The model under review builds one solid part; all positions refer to its coordinate system, in mm. A direction names the side the tool comes from. Round coordinates to 2 decimals unless told otherwise and drop trailing zeros. Write each loop counter-clockwise with the first axis right and the second up, starting at its lowest first coordinate (ties: lowest second). Pieces come first, ordered by that corner, then holes. Notation, with made-up numbers: M 29,-2.75 L 58,-2.75 A13 cw 58,5.25 Z; hole C 12,40.25 d1. An arc over 180 degrees is marked long. Write item = value, one per line. Start each with the question number.
Item 1: Tool access review of faces 1 (the flat face through (-32, 0, -6.35)), 2 (the flat face through (32, 0, -19.05)), 3 (the flat face through (-31.572, -5.474, -15.919)): name each direction out of +Z, -Z, +X, -X, +Y, -Y from which nothing blocks a thin tool from reaching the whole face with its end or side.
Item 2: Take a section at A-A, the plane x = 30. Give the boundary of the cut face in (y, z), plus the area to 3 significant figures.
Item 3: Take a section at C-C, the plane z = 6.5. Give the boundary of the cut face in (x, y).
Item 4: Take a section at B-B, the plane z = 19.5. Give the boundary of the cut face in (x, y), plus the area to 3 significant figures.
Item 5: The part is to be moulded in two halves that separate along X. For faces 4 (the flat face through (-12.26, -0.27, 9.7)), 5 (the flat face through (31.572, 5.474, -9.481)), 6 (the flat face through (0, 0, 25.4)), say which applies: +X half, -X half, draft (parallel to the pull), parting line (faces both ways), or undercut.
Item 6: To check wall thickness, follow line 1 along X through (y, z) = (-13, -19); line 2 along X through (y, z) = (10.5, -20); line 3 along X through (y, z) = (16.5, -6.5). State the ranges of each line that lie inside material, in increasing order.
Item 7: For pin 1 Ø3.5 at (x, y) = (26, 0.5) entering from +Z; pin 2 Ø6 at (x, y) = (-35.5, 1) entering from -Z; pin 3 Ø1 at (y, z) = (3.5, 4.5) entering from +X; pin 4 Ø12 at (x, z) = (-27, 7) entering from -Y (3 decimals), all flat-tipped, find the tip position at first contact; note any pin that passes through.
from build123d import *

# Parameters (mm, degrees)
F0_W      = 38.1
F0_H      = 38.1
F1_DEPTH  = 25.4
F1_TAPER  = 35
F2_DEPTH  = 25.4
F2_FACE_W = 38.1
F2_FACE_H = 38.1
F3_DEPTH  = 25.4
F3_TAPER  = 35
F7_DEPTH  = 25.4
F9_R      = 0.127
F10_DEPTH = 25.4


with BuildPart() as f1:
    # F0 (on Top) → F1 (new body)
    with BuildSketch(Plane.XY):
        Rectangle(F0_W, F0_H)
    extrude(amount=F1_DEPTH, taper=F1_TAPER)

    # F2 (add): a face of the model
    f2_faces = [f1.faces().sort_by_distance(p)[0] for p in [
        (0, 0, 0),
    ]]
    extrude(f2_faces, amount=F2_DEPTH)

    # F2_face (on face) → F3 (cut)
    with BuildSketch(Plane(origin=(0, 0, -25.4), x_dir=(1, 0, 0), z_dir=(0, 0, -1))):
        Rectangle(F2_FACE_W, F2_FACE_H)
    extrude(amount=-F3_DEPTH, taper=F3_TAPER, mode=Mode.SUBTRACT)

    # F6 (on face) → F7 (join)
    with BuildSketch(Plane(origin=(-19.05, 0, 0), x_dir=(0, -1, 0), z_dir=(-1, 0, 0))):
        Polygon((3.6661742094, -6.35), (-3.6661742094, -6.35), (-7.3323484187, -12.7), (-3.6661742094, -19.05), (3.6661742094, -19.05), (7.3323484187, -12.7), align=None)
    extrude(amount=F7_DEPTH)

    # F8: F1 across plane


with BuildPart() as f1_1:
    add(f1.part)
    add(f1.part.mirror(Plane.YZ))

    # F9 (on face) → F10 (join)
    with BuildSketch(Plane.XY.offset(25.4)):
        with Locations((0, 0.889)):
            Circle(F9_R)
        with Locations((-0.4445, 0.769896584)):
            Circle(F9_R)
        with Locations((-0.769896584, 0.4445)):
            Circle(F9_R)
        with Locations((-0.889, 0)):
            Circle(F9_R)
        with Locations((-0.769896584, -0.4445)):
            Circle(F9_R)
        with Locations((-0.4445, -0.769896584)):
            Circle(F9_R)
        with Locations((0, -0.889)):
            Circle(F9_R)
        with Locations((0.4445, -0.769896584)):
            Circle(F9_R)
        with Locations((0.769896584, -0.4445)):
            Circle(F9_R)
        with Locations((0.889, 0)):
            Circle(F9_R)
        with Locations((0.769896584, 0.4445)):
            Circle(F9_R)
        with Locations((0.4445, 0.769896584)):
            Circle(F9_R)
    extrude(amount=F10_DEPTH)


solid = f1_1.part
Response values:
q1.face_1 = +Z, -X, +Y, -Y
q1.face_2 = -Z, +X, +Y, -Y
q1.face_3 = -Z, -X, -Y
q2.outline = M -7.33,-12.7 L -3.67,-19.05 L 3.67,-19.05 L 7.33,-12.7 L 3.67,-6.35 L -3.67,-6.35 Z
q2.area = 140 mm2
q3.outline = M -14.5,-14.5 L 14.5,-14.5 L 14.5,14.5 L -14.5,14.5 Z
q4.outline = M -5.4,-5.4 L 5.4,-5.4 L 5.4,5.4 L -5.4,5.4 Z
q4.area = 116 mm2
q5.face_4 = -X half
q5.face_5 = draft
q5.face_6 = undercut
q6.line_1 = -19.05 to -14.57, 14.57 to 19.05
q6.line_2 = -19.05 to -15.27, 15.27 to 19.05
q6.line_3 = -19.05 to 19.05
q7.pin_1 = -6.35
q7.pin_2 = -19.05
q7.pin_3 = 16.25
q7.pin_4 = through
